from build123d import *

# Parameters (mm, degrees)
SKETCH_1_R          = 2
EXTRUDE_1_DEPTH     = 2
CUT_EXTRUDE_1_DEPTH = 30.908699941


with BuildPart() as part:
    # 草图1 → 凸台-拉伸1 (new body)
    with BuildSketch(Plane(origin=(0, 0, 0), x_dir=(1, 0, 0), z_dir=(0, 1, 0))):
        Polygon((-19.887274719, -20.85738568), (19.887274719, -20.85738568), (21.342441161, -19.402219238), (21.342441161, 19.402219238), (19.887274719, 20.85738568), (-19.887274719, 20.85738568), (-21.342441161, 19.402219238), (-21.342441161, -19.402219238), align=None)
        with Locations(Location((15.25, 15.25, 0), (0, 0, 270))):
            Circle(SKETCH_1_R, mode=Mode.SUBTRACT)
        with Locations(Location((-15.25, 15.25, 0), (0, 0, 90))):
            Circle(SKETCH_1_R, mode=Mode.SUBTRACT)
        with Locations(Location((15.25, -15.25, 0), (0, 0, 90))):
            Circle(SKETCH_1_R, mode=Mode.SUBTRACT)
        with Locations(Location((-15.25, -15.25, 0), (0, 0, 270))):
            Circle(SKETCH_1_R, mode=Mode.SUBTRACT)
    extrude(amount=EXTRUDE_1_DEPTH)

    # 草图2 → 切除-拉伸1 (cut, through all)
    with BuildSketch(Plane(origin=(0, 2, 0), x_dir=(1, 0, 0), z_dir=(0, 1, 0))):
        with BuildLine():
            Line((-19.842796432, 12.473949701), (-21.342441161, 12.473949701))
            Line((-21.342441161, 12.473949701), (-21.342441161, 20.85738568))
            Line((-21.342441161, 20.85738568), (-7.423925003, 20.85738568))
            Line((-7.423925003, 20.85738568), (-9.313125328, 18.968185355))
            Line((-9.313125328, 18.968185355), (-14.512267744, 18.968185355))
            ThreePointArc((-14.512267744, 18.968185355), (-18.522532331, 16.825056167), (-19.842796432, 12.473949701))
        make_face()
        with BuildLine():
            Line((7.423925003, 20.85738568), (21.342441161, 20.85738568))
            Line((21.342441161, 20.85738568), (21.342441161, 12.473949701))
            Line((21.342441161, 12.473949701), (19.842796432, 12.473949701))
            ThreePointArc((19.842796432, 12.473949701), (18.522532331, 16.825056167), (14.512267744, 18.968185355))
            Line((14.512267744, 18.968185355), (9.313125328, 18.968185355))
            Line((9.313125328, 18.968185355), (7.423925003, 20.85738568))
        make_face()
        with BuildLine():
            Line((9.313125328, -18.968185355), (7.423925003, -20.85738568))
            Line((7.423925003, -20.85738568), (21.342441161, -20.85738568))
            Line((21.342441161, -20.85738568), (21.342441161, -12.473949701))
            Line((21.342441161, -12.473949701), (19.842796432, -12.473949701))
            ThreePointArc((19.842796432, -12.473949701), (18.522532331, -16.825056167), (14.512267744, -18.968185355))
            Line((14.512267744, -18.968185355), (9.313125328, -18.968185355))
        make_face()
        with BuildLine():
            Line((-7.423925003, -20.85738568), (-21.342441161, -20.85738568))
            Line((-21.342441161, -20.85738568), (-21.342441161, -12.473949701))
            Line((-21.342441161, -12.473949701), (-19.842796432, -12.473949701))
            ThreePointArc((-19.842796432, -12.473949701), (-18.522532331, -16.825056167), (-14.512267744, -18.968185355))
            Line((-14.512267744, -18.968185355), (-9.313125328, -18.968185355))
            Line((-9.313125328, -18.968185355), (-7.423925003, -20.85738568))
        make_face()
    extrude(amount=-CUT_EXTRUDE_1_DEPTH, mode=Mode.SUBTRACT)


solid = part.part
Work out the finished part from the listing and answer in its coordinate system (mm). A direction names the side the tool comes from. Give positions to 0.01 mm unless a question says otherwise; leave off trailing zeros. Loops run counter-clockwise (first coordinate to the right, second up) from the corner with the lowest first, then second, coordinate; pieces in that order, holes last. Notation, with made-up numbers: (6, 12.25) - (30, 12.25) arc R11 cw to (30, 31.25) - close; hole circle Ø10 at (53.25, 43.25). An arc over 180 degrees is marked (long way). Answer in a Markdown table with one row per item.
(1) Flat-ended cylindrical pins translate along their axes: pin 1 Ø1 at (x, y) = (10.5, 0.5) entering from -Z; pin 2 Ø0.7 at (x, y) = (20.5, 1) entering from -Z; pin 3 Ø5 at (x, z) = (-15.25, 15.25) entering from -Y; pin 4 Ø1.2 at (x, y) = (21, 0.5) entering from +Z. Find the tip coordinate at first contact, or state that the pin passes through.
Results list:
| item | result |
|---|---|
| pin 1 | stops at z = -18.97 |
| pin 2 | stops at z = -12.47 |
| pin 3 | stops at y = 0 |
| pin 4 | stops at z = 12.47 |
(2) A tool of negligible diameter and unlimited length cuts with its end or side. For faces 5 (the face through (-21.342, 1, 0)), 6 (the face through (12, 1, 18.968)), 7 (the face through (12, 1, -18.968)), from which of +Z, -Z, +X, -X, +Y, -Y can it reach the whole face along a straight path? Write none if from no direction.
Results list:
| item | result |
|---|---|
| face 5 | +Z, -Z, -X, +Y, -Y |
| face 6 | +Z, +X, +Y, -Y |
| face 7 | -Z, +X, +Y, -Y |
(3) Section C-C (x = 16) is taken. Give the vertices of the cut face in (y, z).
Results list:
| item | result |
|---|---|
| outline | (0, -18.62) - (2, -18.62) - (2, -17.1) - (0, -17.1) - close; (0, -13.4) - (2, -13.4) - (2, 13.4) - (0, 13.4) - close; (0, 17.1) - (2, 17.1) - (2, 18.62) - (0, 18.62) - close |
(4) Section B-B (z = -15.25) is taken. Give the vertices of the cut face in (x, y).
Results list:
| item | result |
|---|---|
| outline | (-19.45, 0) - (-17.25, 0) - (-17.25, 2) - (-19.45, 2) - close; (-13.25, 0) - (13.25, 0) - (13.25, 2) - (-13.25, 2) - close; (17.25, 0) - (19.45, 0) - (19.45, 2) - (17.25, 2) - close |
(5) Section A-A (y = 1.15) is taken. Give the vertices of the cut face in (x, z).
Results list:
| item | result |
|---|---|
| outline | (-21.34, -12.47) - (-19.84, -12.47) arc R5.94 ccw to (-14.51, -18.97) - (-9.31, -18.97) - (-7.42, -20.86) - (7.42, -20.86) - (9.31, -18.97) - (14.51, -18.97) arc R5.94 ccw to (19.84, -12.47) - (21.34, -12.47) - (21.34, 12.47) - (19.84, 12.47) arc R5.94 ccw to (14.51, 18.97) - (9.31, 18.97) - (7.42, 20.86) - (-7.42, 20.86) - (-9.31, 18.97) - (-14.51, 18.97) arc R5.94 ccw to (-19.84, 12.47) - (-21.34, 12.47) - close; hole circle Ø4 at (-15.25, -15.25); hole circle Ø4 at (-15.25, 15.25); hole circle Ø4 at (15.25, -15.25); hole circle Ø4 at (15.25, 15.25) |
(6) Consider L1, parallel to X at y = 0.55, z = 15.25; L2, parallel to X at y = 0.2, z = 16.5; L3, parallel to Z at x = 16.5, y = 1.8. Determine where each line is inside the solid, lowest interval first. Write a range as [from, to].
Results list:
| item | result |
|---|---|
| L1 | x = [-19.45, -17.25], [-13.25, 13.25], [17.25, 19.45] |
| L2 | x = [-18.77, -16.81], [-13.69, 13.69], [16.81, 18.77] |
| L3 | z = [-18.41, -16.81], [-13.69, 13.69], [16.81, 18.41] |
(7) Section D-D (x = 11.5) is taken. Give the vertices of the cut face in (y, z).
Results list:
| item | result |
|---|---|
| outline | (0, -18.97) - (2, -18.97) - (2, 18.97) - (0, 18.97) - close |
(8) For a pull along Z with two mould halves and no side action, classify faces 1 (the face through (0, 1, -20.857)), 2 (the face through (0, 2, 0)), 3 (the face through (-17.233, 0.986, -14.99)), 4 (the face through (17.233, 0.986, -15.51)) as pulls with the +Z half, pulls with the -Z half, needs draft (parallel to the pull), parting line crosses it, or undercut.
Results list:
| item | result |
|---|---|
| face 1 | pulls with the -Z half |
| face 2 | needs draft |
| face 3 | undercut |
| face 4 | undercut |
